Could you check a few things on this model? Use its own coordinates, in mm. Face numbers are marked on the shaded views. A direction names the side the tool comes from. Round coordinates to 2 decimals unless told otherwise and drop trailing zeros. Write each loop counter-clockwise with the first axis right and the second up, starting at its lowest first coordinate (ties: lowest second). Pieces come first, ordered by that corner, then holes. Notation, with made-up numbers: M -10.5,88 L -4.5,88 A27 ccw -4.5,104 Z; hole C 30,80 d7. An arc over 180 degrees is marked long. One line per item, written item: value. Start each with the question number.
(1) I want a section at C-C on y = 153. Please give me the cut outline in (x, z), and give its area (3 significant figures).
(2) I'm going to push flat-ended pins straight in: pin 1 Ø3 at (x, y) = (356.5, -55.5) entering from +Z; pin 2 Ø3 at (x, z) = (322.5, 325) entering from -Y; pin 3 Ø5 at (x, z) = (-44, 184) entering from -Y. Where does each tip first touch, or does it pass through?
(3) I want a section at B-B on x = 363.5. Please give me the cut outline in (y, z).
(4) Thinking about a two-plate mould opening in X: for the marked faces 1, 2, 3 and 4, which applies, released by +X, released by -X, zero draft, split by the parting line, or undercut?
(5) Which directions (+Z, -Z, +X, -X, +Y, -Y) give clear straight access to the entire face, cutting with the end or side of a thin tool? Please do the marked faces 5 and 6.
(6) If I drill on L1, parallel to X at y = 127, z = 136; L2, parallel to Z at x = 67, y = 194.5; L3, parallel to Y at x = 16, z = 66, over which ranges is the centre line in solid material (lowest first)?
(7) I want a section at D-D on y = -95.5. Please give me the cut outline in (x, z).
(8) I want a section at A-A on z = 185. Please give me the cut outline in (x, y), and give its area (3 significant figures).
```python
from build123d import *

# Parameters (mm, degrees)
F0_W     = 533.4
F0_H     = 304.8
F1_DEPTH = 381
F2_T     = -6.35
F3_W     = 527.05
F3_H     = 6.35
F4_DEPTH = 76.2


with BuildPart() as f1:
    # F0 (on Top) → F1 (new body)
    with BuildSketch(Plane.XY):
        with Locations((219.900687, 92.017783)):
            Rectangle(F0_W, F0_H)
    extrude(amount=F1_DEPTH)

    # F2
    f2_openings = [f1.faces().sort_by_distance(p)[0] for p in [
        (219.900687, 92.017783, 381),
        (219.900687, -60.382217, 190.5),
    ]]
    offset(amount=F2_T, openings=f2_openings)

    # F3 (on face) → F4 (join)
    with BuildSketch(Plane.XZ.offset(60.382217)):
        with Locations((216.725687, 3.175)):
            Rectangle(F3_W, F3_H)
    extrude(amount=F4_DEPTH)


solid = f1.part
```
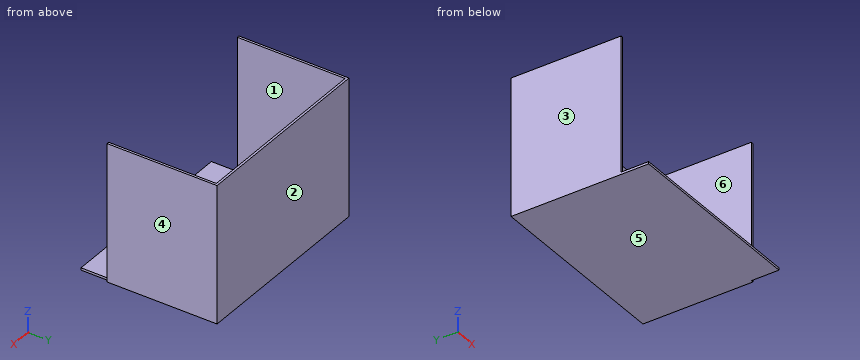
Found:
1. outline: M -46.8,0 L 486.6,0 L 486.6,381 L 480.25,381 L 480.25,6.35 L -40.45,6.35 L -40.45,381 L -46.8,381 Z
1. area: 8,150 mm²
2. pin 1: stops at z = 6.35
2. pin 2: stops at y = 238.07
2. pin 3: stops at y = -60.38
3. outline: M -136.58,0 L 244.42,0 L 244.42,381 L 238.07,381 L 238.07,6.35 L -136.58,6.35 Z
4. face 1: undercut
4. face 2: zero draft
4. face 3: released by -X
4. face 4: released by +X
5. face 5: -Z, +X, -X, +Y, -Y
5. face 6: +Z, -Y
6. L1: x = -46.8 to -40.45, 480.25 to 486.6
6. L2: z = 0 to 6.35
6. L3: y = 238.07 to 244.42
7. outline: M -46.8,0 L 480.25,0 L 480.25,6.35 L -46.8,6.35 Z
8. outline: M -46.8,-60.38 L -40.45,-60.38 L -40.45,238.07 L 480.25,238.07 L 480.25,-60.38 L 486.6,-60.38 L 486.6,244.42 L -46.8,244.42 Z
8. area: 7,180 mm²
